Input: part model. Units: mm. Frame: model coordinates. A direction names the side the tool comes from. Round coordinates to 2 decimals unless told otherwise and drop trailing zeros. Write each loop counter-clockwise with the first axis right and the second up, starting at its lowest first coordinate (ties: lowest second). Pieces come first, ordered by that corner, then holes. Notation, with made-up numbers: (46, 46.25) -> (100, 46.25) arc R13 cw to (100, 60.25) -> close; hole circle Ø1 at (-36, 7). An arc over 180 degrees is marked (long way). Write item = value, one per line.
```python
from build123d import *

# Parameters (mm, degrees)
SKETCH_1_R          = 3.5
EXTRUDE_1_DEPTH     = 63
SKETCH_2_R          = 5.249939155
SKETCH_2_R_2        = 3
CUT_EXTRUDE_1_DEPTH = 6
SKETCH_3_R          = 5.960650936
SKETCH_3_R_2        = 3
CUT_EXTRUDE_2_DEPTH = 6


with BuildPart() as part:
    # ｽｹｯﾁ1 → ﾎﾞｽ - 押し出し1 (new body)
    with BuildSketch(Plane.XY):
        Circle(SKETCH_1_R)
    extrude(amount=EXTRUDE_1_DEPTH)

    # ｽｹｯﾁ2 → ｶｯﾄ - 押し出し1 (cut)
    with BuildSketch(Plane.XY.offset(63)):
        Circle(SKETCH_2_R)
        Circle(SKETCH_2_R_2, mode=Mode.SUBTRACT)
    extrude(amount=-CUT_EXTRUDE_1_DEPTH, mode=Mode.SUBTRACT)

    # ｽｹｯﾁ3 → ｶｯﾄ - 押し出し2 (cut)
    with BuildSketch(Plane(origin=(0, 0, 0), x_dir=(-1, 0, 0), z_dir=(0, 0, -1))):
        Circle(SKETCH_3_R)
        Circle(SKETCH_3_R_2, mode=Mode.SUBTRACT)
    extrude(amount=-CUT_EXTRUDE_2_DEPTH, mode=Mode.SUBTRACT)


solid = part.part
```
1) Cut plane C-C (z = 35). Return the cut outline in (x, y), and give its area (3 significant figures).
Solutions:
outline = circle Ø7 at (0, 0)
area = 38.5 mm^2
2) Cut plane B-B (y = 0.75). Return the cut outline in (x, z).
Solutions:
outline = (-3.42, 6) -> (-2.9, 6) -> (-2.9, 0) -> (2.9, 0) -> (2.9, 6) -> (3.42, 6) -> (3.42, 57) -> (2.9, 57) -> (2.9, 63) -> (-2.9, 63) -> (-2.9, 57) -> (-3.42, 57) -> close
3) First-contact query: P1, Ø1.5, axis at y = 1, z = 17, coming from the +X side; P2, Ø1, axis at y = 2, z = 20, coming from the -X side. Flat tips, straight axial feed; report the tip coordinate or a pass-through.
Solutions:
P1 = 3.49
P2 = -3.16
4) Access query for faces 1 (the face through (3, 0, 3)), 2 (the face through (-3, 0, 60)), 3 (the face through (3.233, -1.341, 31.143)). Directions: +Z, -Z, +X, -X, +Y, -Y. A direction counts if a zero-diameter tool reaches every point of the face in a straight line with its end or side. Return the directions, or none.
Solutions:
face_1 = -Z
face_2 = +Z
face_3 = +Z, -Z
5) Cut plane A-A (x = 0). Return the cut outline in (y, z), and give its area (3 significant figures).
Solutions:
outline = (-3.5, 6) -> (-3, 6) -> (-3, 0) -> (3, 0) -> (3, 6) -> (3.5, 6) -> (3.5, 57) -> (3, 57) -> (3, 63) -> (-3, 63) -> (-3, 57) -> (-3.5, 57) -> close
area = 429 mm^2
6) Line query: L1, parallel to X at y = 0.25, z = 25.5; L2, parallel to Z at x = -1.75, y = 2.75. Output: solid intervals per line, ascending. Write a range as from..to.
Solutions:
L1 = -3.49..3.49
L2 = 6..57
